```python
from build123d import *

# Parameters (mm, degrees)
F1_DEPTH = 4


with BuildPart() as f1:
    # F0 (on Top) → F1 (new body, symmetric)
    with BuildSketch(Plane.XY):
        with BuildLine():
            Line((-3.245455, 16.687331), (-29.743182, 11.533891))
            ThreePointArc((-29.743182, 11.533891), (-39.25, 0), (-29.743182, -11.533891))
            Line((-29.743182, -11.533891), (-3.245455, -16.687331))
            ThreePointArc((-3.245455, -16.687331), (-1.630241, -16.921652), (0, -17))
            ThreePointArc((0, -17), (1.630241, -16.921652), (3.245455, -16.687331))
            Line((3.245455, -16.687331), (29.743182, -11.533891))
            ThreePointArc((29.743182, -11.533891), (39.25, 0), (29.743182, 11.533891))
            Line((29.743182, 11.533891), (3.245455, 16.687331))
            ThreePointArc((3.245455, 16.687331), (1.630241, 16.921652), (0, 17))
            ThreePointArc((0, 17), (-1.630241, 16.921652), (-3.245455, 16.687331))
        make_face()
        Polygon((-27.5, -10.854185), (-36.9, -5.427093), (-36.9, 5.427093), (-27.5, 10.854185), (-18.1, 5.427093), (-18.1, -5.427093), align=None, mode=Mode.SUBTRACT)
        with BuildLine():
            ThreePointArc((0, -15.975), (-15.975, 0), (0, 15.975))
            ThreePointArc((0, 15.975), (15.975, 0), (0, -15.975))
        make_face(mode=Mode.SUBTRACT)
        Polygon((27.5, 10.854185), (36.9, 5.427093), (36.9, -5.427093), (27.5, -10.854185), (18.1, -5.427093), (18.1, 5.427093), align=None, mode=Mode.SUBTRACT)
    extrude(amount=F1_DEPTH, both=True)


solid = f1.part
```
For this review, take the finished solid that the model builds, in its own axes (mm). A direction names the side the tool comes from. Coordinates: 2 decimals unless noted, no trailing zeros. Write each loop counter-clockwise with the first axis right and the second up, starting at its lowest first coordinate (ties: lowest second). Pieces come first, ordered by that corner, then holes. Notation, with made-up numbers: (54.25, 35) - (69.25, 35) arc R16 cw to (69.25, 55) - close; hole circle Ø6 at (-14, -14.5). An arc over 180 degrees is marked (long way). Answer in a Markdown table with one row per item. Add a question column.
Q1. Draft analysis for pull direction Y (two halves, no side actions). For faces 1 (the cylindrical face through (39.248, -0.227, 0.056)), 2 (the flat face through (16.68, 14.075, 0.056)), 3 (the flat face through (-15, 6, 4)), 4 (the flat face through (-32.1, -8.2, 0.1)), state which applies: +Y half, -Y half, draft (parallel to the pull), parting line (faces both ways), or undercut.
Q2. We need section D-D, the plane x = 12. State the section outline as (y, z) points.
Q3. Tool access review of faces 5 (the flat face through (-16.309, 14.147, 0.056)), 6 (the flat face through (22.9, -8.2, 0.1)): name each direction out of +Z, -Z, +X, -X, +Y, -Y from which nothing blocks a thin tool from reaching the whole face with its end or side.
Q4. We need section B-B, the plane y = 0. State the section outline as (x, z) points (3 decimals), and give its area (3 significant figures).
Q5. We need section C-C, the plane x = -11.5. State the section outline as (y, z) points, and give its area (3 significant figures).
Q6. We need section A-A, the plane z = 3. State the section outline as (x, y) points (3 decimals).
Q7. For P1, Ø4, axis at y = 2.5, z = -2, coming from the +X side; P2, Ø4, axis at y = -9.5, z = 3, coming from the -X side (3 decimals); P3, Ø3, axis at x = -12.5, z = 0.5, coming from the +Y side, all flat-tipped, find the tip position at first contact; note any pin that passes through.
Q8. For probe 1 along X at (y, z) = (10, 0.25); probe 2 along X at (y, z) = (-5.5, 1.75); probe 3 along Y at (x, z) = (14.5, -2.75), list the stretches that pass through material, from the lowest coordinate up.
Answer list:
| question | item | result |
|---|---|---|
| 1 | face 1 | parting line |
| 1 | face 2 | +Y half |
| 1 | face 3 | draft |
| 1 | face 4 | undercut |
| 2 | outline | (-14.98, -4) - (-10.55, -4) - (-10.55, 4) - (-14.98, 4) - close; (10.55, -4) - (14.98, -4) - (14.98, 4) - (10.55, 4) - close |
| 3 | face 5 | +Z, -Z, -X, +Y |
| 3 | face 6 | +Z, -Z |
| 4 | outline | (-39.25, -4) - (-36.9, -4) - (-36.9, 4) - (-39.25, 4) - close; (-18.1, -4) - (-15.975, -4) - (-15.975, 4) - (-18.1, 4) - close; (15.975, -4) - (18.1, -4) - (18.1, 4) - (15.975, 4) - close; (36.9, -4) - (39.25, -4) - (39.25, 4) - (36.9, 4) - close |
| 4 | area | 71.6 mm2 |
| 5 | outline | (-15.08, -4) - (-11.09, -4) - (-11.09, 4) - (-15.08, 4) - close; (11.09, -4) - (15.08, -4) - (15.08, 4) - (11.09, 4) - close |
| 5 | area | 63.9 mm2 |
| 6 | outline | (-29.743, -11.534) - (-3.245, -16.687) arc R17 ccw to (0, -17) arc R17 ccw to (3.245, -16.687) - (29.743, -11.534) arc R11.75 ccw to (29.743, 11.534) - (3.245, 16.687) arc R17 ccw to (0, 17) arc R17 ccw to (-3.245, 16.687) - (-29.743, 11.534) arc R11.75 ccw to start; hole (-36.9, -5.427) - (-27.5, -10.854) - (-18.1, -5.427) - (-18.1, 5.427) - (-27.5, 10.854) - (-36.9, 5.427) - close; hole circle Ø31.95 at (0, 0); hole (18.1, -5.427) - (27.5, -10.854) - (36.9, -5.427) - (36.9, 5.427) - (27.5, 10.854) - (18.1, 5.427) - close |
| 7 | P1 | stops at x = 39.24 |
| 7 | P2 | stops at x = -36.545 |
| 7 | P3 | stops at y = 15.18 |
| 8 | probe 1 | x = -33.67 to -28.98, -26.02 to -12.46, 12.46 to 26.02, 28.98 to 33.67 |
| 8 | probe 2 | x = -37.88 to -36.77, -18.23 to -15, 15 to 18.23, 36.77 to 37.88 |
| 8 | probe 3 | y = -14.5 to -6.7, 6.7 to 14.5 |
